Read the model definition and answer for the solid it produces. Units are mm, in the model's axes. A direction names the side the tool comes from. Round coordinates to 2 decimals unless told otherwise and drop trailing zeros. Write each loop counter-clockwise with the first axis right and the second up, starting at its lowest first coordinate (ties: lowest second). Pieces come first, ordered by that corner, then holes. Notation, with made-up numbers: (29.5, -2.75) -> (76.5, -2.75) arc R19 ccw to (76.5, 31.25) -> close; hole circle Ø5 at (72, 31.5). An arc over 180 degrees is marked (long way). Return JSON: item names as keys, results as strings.
from build123d import *

# Parameters (mm, degrees)
SKETCH1_R                       = 1.016
BOSS_EXTRUDE1_DEPTH             = 2
SKETCH2_R                       = 4.7
BOSS_EXTRUDE2_DEPTH             = 3
BOSS_EXTRUDE5_DEPTH             = 8
BOSS_EXTRUDE6_REACH             = 45.704
BOSS_EXTRUDE6_DIRECTION_2_REACH = 45.704
SKETCH4_W                       = 22.5
SKETCH4_H                       = 14.127681706
CUT_EXTRUDE1_DEPTH              = 7
SKETCH5_R                       = 2.5
BOSS_EXTRUDE7_DEPTH             = 1


with BuildPart() as part:
    # Sketch1 → Boss-Extrude1 (new body)
    # profile 1 of 4: a face of its own
    with BuildSketch(Plane.XY):
        with BuildLine():
            Line((-16.05, 5.25), (-16.05, -5.25))
            ThreePointArc((-16.05, -5.25), (-15.801040764, -5.851040764), (-15.2, -6.1))
            Line((-15.2, -6.1), (-11.25, -6.1))
            Line((-11.25, -6.1), (-11.25, 6.1))
            Line((-11.25, 6.1), (-15.2, 6.1))
            ThreePointArc((-15.2, 6.1), (-15.801040764, 5.851040764), (-16.05, 5.25))
        make_face()
        with Locations((-13.9, 0)):
            Circle(SKETCH1_R, mode=Mode.SUBTRACT)
    # profile 2 of 4: a face of its own
    with BuildSketch(Plane.XY):
        with BuildLine():
            Line((16.05, 5.25), (16.05, -5.25))
            ThreePointArc((16.05, -5.25), (15.801040764, -5.851040764), (15.2, -6.1))
            Line((15.2, -6.1), (11.25, -6.1))
            Line((11.25, -6.1), (11.25, 6.094097151))
            Line((11.25, 6.094097151), (15.2, 6.1))
            ThreePointArc((15.2, 6.1), (15.801040764, 5.851040764), (16.05, 5.25))
        make_face()
        with Locations((13.9, 0)):
            Circle(SKETCH1_R, mode=Mode.SUBTRACT)
    # profile 3 of 4: a face of its own
    with BuildSketch(Plane.XY):
        with BuildLine():
            ThreePointArc((15.2, -6.1), (15.801040764, -5.851040764), (16.05, -5.25))
            Line((16.05, -5.25), (16.05, -6.1))
            Line((16.05, -6.1), (15.2, -6.1))
        make_face()
    # profile 4 of 4: a face of its own
    with BuildSketch(Plane.XY):
        with BuildLine():
            ThreePointArc((-16.05, -5.25), (-15.801040764, -5.851040764), (-15.2, -6.1))
            Line((-15.2, -6.1), (-16.05, -6.1))
            Line((-16.05, -6.1), (-16.05, -5.25))
        make_face()
    extrude(amount=BOSS_EXTRUDE1_DEPTH)

    # Sketch2 → Boss-Extrude2 (add)
    with BuildSketch(Plane.XZ.offset(6.1)):
        Polygon((16.05, 2), (11.25, 2), (11.25, 12.784507897), (-1.65, 9.925449639), (-1.65, 2), (-16.05, 2), (-16.05, 0), (-1.65, 0), (-1.65, -30.41033757), (11.25, -31.079190458), (11.25, 0), (16.05, 0), align=None)
        with Locations((4.75, -19)):
            Circle(SKETCH2_R, mode=Mode.SUBTRACT)
    extrude(amount=BOSS_EXTRUDE2_DEPTH)

    # Sketch2<3> → Boss-Extrude5 (add)
    with BuildSketch(Plane.XZ.offset(6.1)):
        with BuildLine():
            Line((11.201492875, 11.3190285), (11.25, 11.337476622))
            Line((11.25, 11.337476622), (11.25, 12.784507897))
            Line((11.25, 12.784507897), (-1.65, 9.925449639))
            Line((-1.65, 9.925449639), (-1.65, 7.134527797))
            ThreePointArc((-1.65, 7.134527797), (0.2068653, 8.32459199), (2.276136625, 9.087689437))
            Line((2.276136625, 9.087689437), (11.201492875, 11.3190285))
        make_face()
        with BuildLine():
            ThreePointArc((4.75, -29.2), (1.356725547, -28.619027419), (-1.65, -26.942291861))
            Line((-1.65, -26.942291861), (-1.65, -30.41033757))
            Line((-1.65, -30.41033757), (11.25, -31.079190458))
            Line((11.25, -31.079190458), (11.25, -29.090542554))
            ThreePointArc((11.25, -29.090542554), (10.201413429, -29.172617079), (9.149976222, -29.2))
            Line((9.149976222, -29.2), (4.75, -29.2))
        make_face()
    extrude(amount=BOSS_EXTRUDE5_DEPTH)

    # Boss-Extrude6: up to this face of the body (flat: up to its plane)
    boss_extrude6_end = Plane(part.part.faces().sort_by_distance((16.05, -1.925, 1))[0])
    # Sketch3 → Boss-Extrude6 (add, up to the picked face)
    with BuildSketch(Plane(origin=(11.25, 0, 0), x_dir=(0, 0, -1), z_dir=(1, 0, 0)), mode=Mode.PRIVATE) as boss_extrude6_sk1:
        Polygon((-7.665828596, -9.1), (-2, -3.457464127), (-2, -9.1), align=None)
    boss_extrude6_tool1 = split(extrude(boss_extrude6_sk1.sketch, amount=BOSS_EXTRUDE6_REACH, mode=Mode.PRIVATE), bisect_by=boss_extrude6_end, keep=Keep.BOTH, mode=Mode.PRIVATE)
    add(boss_extrude6_tool1.solids().sort_by(Axis((11.25, -7.219155, 3.88861), (1, 0, 0)))[0])

    # Boss-Extrude6 direction 2: up to this face of the body (flat: up to its plane)
    boss_extrude6_direction_2_end = Plane(part.part.faces().sort_by_distance((-16.05, -1.925, 1))[0])
    # Sketch3 → Boss-Extrude6 direction 2 (add, up to the picked face)
    with BuildSketch(Plane(origin=(11.25, 0, 0), x_dir=(0, 0, -1), z_dir=(1, 0, 0)), mode=Mode.PRIVATE) as boss_extrude6_direction_2_sk1:
        Polygon((-7.665828596, -9.1), (-2, -3.457464127), (-2, -9.1), align=None)
    boss_extrude6_direction_2_tool1 = split(extrude(boss_extrude6_direction_2_sk1.sketch, amount=-BOSS_EXTRUDE6_DIRECTION_2_REACH, mode=Mode.PRIVATE), bisect_by=boss_extrude6_direction_2_end, keep=Keep.BOTH, mode=Mode.PRIVATE)
    add(boss_extrude6_direction_2_tool1.solids().sort_by(Axis((11.25, -7.219155, 3.88861), (-1, 0, 0)))[0])

    # Sketch4 → Cut-Extrude1 (cut)
    with BuildSketch(Plane(origin=(0, -6.1, 0), x_dir=(1, 0, 0), z_dir=(0, 1, 0))):
        with Locations((0, -7.063840853)):
            Rectangle(SKETCH4_W, SKETCH4_H)
    extrude(amount=CUT_EXTRUDE1_DEPTH, mode=Mode.SUBTRACT)

    # Sketch5 → Boss-Extrude7 (add)
    with BuildSketch(Plane.XZ.offset(9.1)):
        with BuildLine():
            Line((-1.65, 0), (-1.65, -26.942291861))
            ThreePointArc((-1.65, -26.942291861), (1.356725547, -28.619027419), (4.75, -29.2))
            Line((4.75, -29.2), (9.149976222, -29.2))
            ThreePointArc((9.149976222, -29.2), (10.201413429, -29.172617079), (11.25, -29.090542554))
            Line((11.25, -29.090542554), (11.25, 0))
            Line((11.25, 0), (16.05, 0))
            Line((16.05, 0), (16.05, 7.665828596))
            Line((16.05, 7.665828596), (11.25, 7.665828596))
            Line((11.25, 7.665828596), (11.25, 11.337476622))
            Line((11.25, 11.337476622), (11.201492875, 11.3190285))
            Line((11.201492875, 11.3190285), (2.276136625, 9.087689437))
            ThreePointArc((2.276136625, 9.087689437), (0.2068653, 8.32459199), (-1.65, 7.134527797))
            Line((-1.65, 7.134527797), (-1.65, 7.665828596))
            Line((-1.65, 7.665828596), (-16.05, 7.665828596))
            Line((-16.05, 7.665828596), (-16.05, 0))
            Line((-16.05, 0), (-1.65, 0))
        make_face()
        with Locations((4.75, -19)):
            Circle(SKETCH5_R, mode=Mode.SUBTRACT)
    extrude(amount=BOSS_EXTRUDE7_DEPTH)


solid = part.part
Item 1: For a pull along Z with two mould halves and no side action, classify faces 1 (the flat face through (14, -2, 0)), 2 (the flat face through (-13.6, 1.4, 2)), 3 (the flat face through (3, -10.1, -9)) as released by +Z, released by -Z, zero draft, split by the parting line, or undercut.
Worked answers:
{"face 1": "released by -Z", "face 2": "released by +Z", "face 3": "undercut"}
Item 2: Section D-D (x = -9) is taken. Give the vertices of the cut face in (y, z).
Worked answers:
{"outline": "(-10.1, 0) -> (-6.1, 0) -> (-6.1, 4.65) -> (-9.1, 7.67) -> (-10.1, 7.67) -> close"}
Item 3: A tool of negligible diameter and unlimited length cuts with its end or side. For faces 4 (the flat face through (11.25, -8, -16)), 5 (the flat face through (-8.7, -9.6, 7.666)), 6 (the cylindrical face through (1.402, -12.072, -28.635)), from which of +Z, -Z, +X, -X, +Y, -Y can it reach the whole face along a straight path? Write none if from no direction.
Worked answers:
{"face 4": "-Z, +X, +Y, -Y", "face 5": "+Z, -X, +Y, -Y", "face 6": "-Y"}
Item 4: Straight lines are drawn through the part: L1, parallel to Y at x = -13.9, z = 1; L2, parallel to Z at x = -2, y = -9.5; L3, parallel to X at y = -4.5, z = 1. For each, find the intervals that lie inside material, in ascending order. Write a range as [from, to].
Worked answers:
{"L1": "y = [-10.1, -1.02], [1.02, 6.1]", "L2": "z = [0, 7.67]", "L3": "x = [-16.05, -11.25], [11.25, 16.05]"}
Item 5: Section B-B (z = -19) is taken. Give the vertices of the cut face in (x, y), then the cut area to 3 significant figures.
Worked answers:
{"outline": "(-1.65, -10.1) -> (2.25, -10.1) -> (2.25, -9.1) -> (0.05, -9.1) -> (0.05, -6.1) -> (-1.65, -6.1) -> close; (7.25, -10.1) -> (11.25, -10.1) -> (11.25, -6.1) -> (9.45, -6.1) -> (9.45, -9.1) -> (7.25, -9.1) -> close", "area": "18.4 mm2"}
Item 6: Section A-A (y = 3) is taken. Give the vertices of the cut face in (x, z), then the cut area to 3 significant figures.
Worked answers:
{"outline": "(-16.05, 0) -> (-11.25, 0) -> (-11.25, 2) -> (-16.05, 2) -> close; (11.25, 0) -> (16.05, 0) -> (16.05, 2) -> (11.25, 2) -> close", "area": "19.2 mm2"}
Item 7: Section C-C (y = 0) is taken. Give the vertices of the cut face in (x, z).
Worked answers:
{"outline": "(-16.05, 0) -> (-14.92, 0) -> (-14.92, 2) -> (-16.05, 2) -> close; (-12.88, 0) -> (-11.25, 0) -> (-11.25, 2) -> (-12.88, 2) -> close; (11.25, 0) -> (12.88, 0) -> (12.88, 2) -> (11.25, 2) -> close; (14.92, 0) -> (16.05, 0) -> (16.05, 2) -> (14.92, 2) -> close"}
Item 8: Flat-ended cylindrical pins translate along their axes: pin 1 (9 mm diameter, centred on y = -9.5, z = -20, fed in from +X); pin 2 (8 mm diameter, centred on x = 4.75, z = -19, fed in from +Y); pin 3 (4 mm diameter, centred on x = 14.5, y = 3, fed in from +Z). Find the tip coordinate at first contact, or state that the pin passes through.
Worked answers:
{"pin 1": "stops at x = 11.25", "pin 2": "stops at y = -9.1", "pin 3": "stops at z = 2"}
